from build123d import *

# Parameters (mm, degrees)
SKETCH1_R           = 1.05
BOSS_EXTRUDE1_DEPTH = 2
SKETCH2_R           = 1
BOSS_EXTRUDE2_DEPTH = 4


with BuildPart() as part:
    # Sketch1 → Boss-Extrude1 (new body)
    with BuildSketch(Plane.XY):
        Polygon((-53.65, -57.3), (-45.65, -57.3), (-45.65, -45.3), (-26.65, -45.3), (-26.65, -30), (-53.65, -30), align=None)
        with Locations((-51.85, -55.5)):
            Circle(SKETCH1_R, mode=Mode.SUBTRACT)
    extrude(amount=BOSS_EXTRUDE1_DEPTH)

    # Sketch2 → Boss-Extrude2 (add)
    with BuildSketch(Plane.XY.offset(2)):
        with Locations((-28.45, -38.7)):
            Circle(SKETCH2_R)
        with Locations((-51.85, -32.1)):
            Circle(SKETCH2_R)
    extrude(amount=-BOSS_EXTRUDE2_DEPTH)


solid = part.part
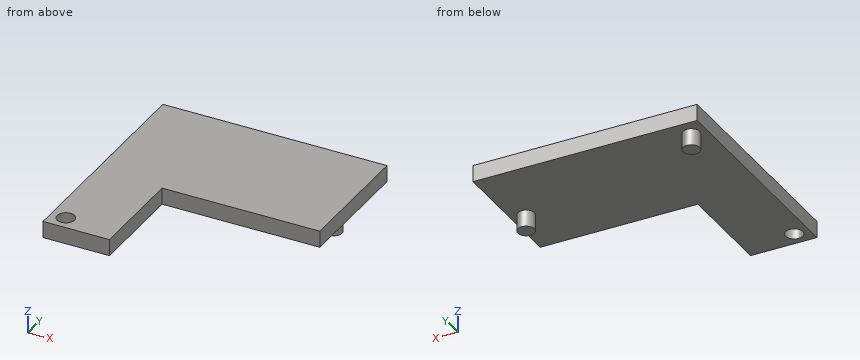
The listing builds one solid part. Answer for the finished solid, in the listing's coordinates (mm). Give positions to 0.01 mm unless a question says otherwise; leave off trailing zeros. Loops run counter-clockwise (first coordinate to the right, second up) from the corner with the lowest first, then second, coordinate; pieces in that order, holes last. Notation, with made-up numbers: M 20.5,0 L 38.5,0 A22 ccw 38.5,15 Z; hole C 67,-24 d7. An arc over 180 degrees is marked long. Answer as CSV lines item,"result".
Item 1: The part is cut by section D-D (z = -0.9). Give the vertices of the cut face in (x, y), and give its area (3 significant figures).
Values follow:
outline,"C -51.85,-32.1 d2; C -28.45,-38.7 d2"
area,"6.28 mm^2"
Item 2: Straight lines are drawn through the part: line 1 along Y through (x, z) = (-51.85, 0.65); line 2 along Y through (x, z) = (-31.75, 1.1); line 3 along Z through (x, y) = (-29.5, -35.25). For each, find the intervals that lie inside material, in ascending order. Write a range as [from, to].
Values follow:
line 1,"y = [-57.3, -56.55], [-54.45, -30]"
line 2,"y = [-45.3, -30]"
line 3,"z = [0, 2]"
Item 3: The part is cut by section C-C (x = -51.85). Give the vertices of the cut face in (y, z), and give its area (3 significant figures).
Values follow:
outline,"M -57.3,0 L -56.55,0 L -56.55,2 L -57.3,2 Z; M -54.45,0 L -33.1,0 L -33.1,-2 L -31.1,-2 L -31.1,0 L -30,0 L -30,2 L -54.45,2 Z"
area,"54.4 mm^2"
Item 4: Given pin 1 Ø1.6 at (y, z) = (-51.5, 0.5) entering from +X; pin 2 Ø4 at (x, y) = (-37, -47.5) entering from -Z (1 decimal); pin 3 Ø1.6 at (x, z) = (-39, 1) entering from -Y; pin 4 Ø2.5 at (x, y) = (-51.85, -55.5) entering from -Z, each flat-ended and moving along its own axis, determine where each tip first touches the part or whether it passes through.
Values follow:
pin 1,"stops at x = -45.65"
pin 2,"passes through"
pin 3,"stops at y = -45.3"
pin 4,"stops at z = 0"
Item 5: The part is cut by section B-B (y = -55.5). Give the vertices of the cut face in (x, z), and give its area (3 significant figures).
Values follow:
outline,"M -53.65,0 L -52.9,0 L -52.9,2 L -53.65,2 Z; M -50.8,0 L -45.65,0 L -45.65,2 L -50.8,2 Z"
area,"11.8 mm^2"
Item 6: The part is cut by section A-A (z = 0.65). Give the vertices of the cut face in (x, y), and give its area (3 significant figures).
Values follow:
outline,"M -53.65,-57.3 L -45.65,-57.3 L -45.65,-45.3 L -26.65,-45.3 L -26.65,-30 L -53.65,-30 Z; hole C -51.85,-55.5 d2.1"
area,"506 mm^2"
